from build123d import *

# Parameters (mm, degrees)
EXTRUDE_1_DEPTH     = 12
SKETCH_2_R          = 1.1
CUT_EXTRUDE_1_DEPTH = 10
SKETCH_3_W          = 4.9
SKETCH_3_H          = 4
CUT_EXTRUDE_2_DEPTH = 1.6
FILLET_1_R          = 4
CUT_EXTRUDE_3_DEPTH = 1


with BuildPart() as part:
    # 草圖1 → 伸長-薄件1 (new body)
    with BuildSketch(Plane.XY):
        Polygon((-12.5, -10), (-6, -10), (-6, 0), (6, 0), (6, -10), (12.5, -10), (12.5, -8.4), (7.6, -8.4), (7.6, 1.6), (-7.6, 1.6), (-7.6, -8.4), (-12.5, -8.4), align=None)
    extrude(amount=EXTRUDE_1_DEPTH)

    # 草圖2 → 除料-伸長1 (cut)
    with BuildSketch(Plane(origin=(0, -8.4, 0), x_dir=(1, 0, 0), z_dir=(0, 1, 0))):
        with Locations(Location((9.5, -4, 0), (0, 0, 270))):
            Circle(SKETCH_2_R)
        with Locations(Location((-9.5, -4, 0), (0, 0, 270))):
            Circle(SKETCH_2_R)
    extrude(amount=-CUT_EXTRUDE_1_DEPTH, mode=Mode.SUBTRACT)

    # 草圖3 → 除料-伸長2 (cut)
    with BuildSketch(Plane.XZ.offset(10)):
        with Locations((-10.05, 10)):
            Rectangle(SKETCH_3_W, SKETCH_3_H)
        with Locations((10.05, 10)):
            Rectangle(SKETCH_3_W, SKETCH_3_H)
    extrude(amount=-CUT_EXTRUDE_2_DEPTH, mode=Mode.SUBTRACT)

    # 圓角1
    fillet_1_edges = [part.edges().sort_by_distance(p)[0] for p in [
        (-12.5, -9.2, 0),
        (-12.5, -9.2, 8),
        (12.5, -9.2, 0),
        (12.5, -9.2, 8),
    ]]
    fillet(fillet_1_edges, radius=FILLET_1_R - 0.0001)  # a hair under: the kernel refuses the full size

    # 草圖4 → 除料-伸長3 (cut)
    with BuildSketch(Plane(origin=(0, -8.4, 0), x_dir=(1, 0, 0), z_dir=(0, 1, 0))):
        Polygon((-7.6, -5.096965511), (-7.6, -2.903034489), (-9.5, -1.806068977), (-11.4, -2.903034489), (-11.4, -5.096965511), (-9.5, -6.193931023), align=None)
        Polygon((7.6, -5.096965511), (9.5, -6.193931023), (11.4, -5.096965511), (11.4, -2.903034489), (9.5, -1.806068977), (7.6, -2.903034489), align=None)
    extrude(amount=-CUT_EXTRUDE_3_DEPTH, mode=Mode.SUBTRACT)


solid = part.part
The model under review builds one solid part; all positions refer to its coordinate system, in mm. A direction names the side the tool comes from. Coordinates: 2 decimals unless noted, no trailing zeros. Loops run counter-clockwise (first coordinate to the right, second up) from the corner with the lowest first, then second, coordinate; pieces in that order, holes last. Notation, with made-up numbers: M 12.5,0 L 62.5,0 A5 cw 62.5,5 Z; hole C 29.5,-35 d8. An arc over 180 degrees is marked long. Put each result on its own line as item: value. Start each with the question number.
Q1. Add section C-C (x = 1.5). Write out the cut boundary in (y, z), and give its area (3 significant figures).
Q2. Add section B-B (z = 11.25). Write out the cut boundary in (x, y), and give its area (3 significant figures).
Q3. Add section D-D (z = 7.75). Write out the cut boundary in (x, y).
Q4. Clearance check with flat-ended pins moving along their axes: pin 1 (2 mm diameter, centred on x = 4, z = 10, fed in from -Y); pin 2 (4 mm diameter, centred on x = 10, z = 4, fed in from +Y); pin 3 (1 mm diameter, centred on y = -0.5, z = 10.5, fed in from -X); pin 4 (1.3 mm diameter, centred on x = 9.5, z = 4, fed in from +Y). State where each tip first meets the part, or that it passes through.
Q5. Add section A-A (y = -8). Write out the cut boundary in (x, z), and give its area (3 significant figures).
Q6. Wall thickness on line 1 (X direction, y = -9.85, z = 4); line 2 (X direction, y = -1, z = 6.5); line 3 (Y direction, x = 5.75, z = 2.25): over which ranges is each line inside the solid? List them lowest first.
Q7. For faces 1 (the cylindrical face through (-9.921, -9.696, 5.016)), 2 (the flat face through (6, -5, 6)), 3 (the flat face through (8, -9, 8)), 4 (the flat face through (-11.4, -9, 4)), list the 3-axis set-ups (+Z, -Z, +X, -X, +Y, -Y) from which the entire face can be reached by the end or side of a thin tool; tool diameter is ignored.
Q8. The part is to be moulded in two halves that separate along X. For faces 5 (the flat face through (12, -8.4, 4)), 6 (the cylindrical face through (11.359, -9.189, 1.203)), 7 (the flat face through (-6, -5, 6)), say which applies: +X half, -X half, draft (parallel to the pull), parting line (faces both ways), or undercut.
Answers:
1. outline: M 0,0 L 1.6,0 L 1.6,12 L 0,12 Z
1. area: 19.2 mm^2
2. outline: M -7.6,-10 L -6,-10 L -6,0 L 6,0 L 6,-10 L 7.6,-10 L 7.6,1.6 L -7.6,1.6 Z
2. area: 56.3 mm^2
3. outline: M -9.89,-10 L -6,-10 L -6,0 L 6,0 L 6,-10 L 9.89,-10 L 9.89,-8.4 L 7.6,-8.4 L 7.6,1.6 L -7.6,1.6 L -7.6,-8.4 L -9.89,-8.4 Z
4. pin 1: stops at y = 0
4. pin 2: stops at y = -8.4
4. pin 3: stops at x = -7.6
4. pin 4: passes through
5. outline: M -7.6,0 L -6,0 L -6,12 L -7.6,12 Z; M 6,0 L 7.6,0 L 7.6,12 L 6,12 Z
5. area: 38.4 mm^2
6. line 1: x = -12.5 to -10.6, -8.4 to -6, 6 to 8.4, 10.6 to 12.5
6. line 2: x = -7.6 to -6, 6 to 7.6
6. line 3: y = 0 to 1.6
7. face 1: +Y, -Y
7. face 2: +Z, -Z, -Y
7. face 3: +Z, +X, +Y, -Y
7. face 4: +Y
8. face 5: draft
8. face 6: +X half
8. face 7: undercut
